from build123d import *

# Parameters (mm, degrees)
F0_R     = 2.5
F1_DEPTH = 5


with BuildPart() as f1:
    # F0 (on Top) → F1 (new body)
    with BuildSketch(Plane.XY):
        with BuildLine():
            ThreePointArc((3.855527, -17.07), (13.669706, -10.926534), (17.5, 0))
            ThreePointArc((17.5, 0), (13.593381, 11.021343), (3.617714, 17.121978))
            ThreePointArc((3.617714, 17.121978), (-0.121713, 17.499577), (-3.855527, 17.07))
            ThreePointArc((-3.855527, 17.07), (-17.499577, -0.121713), (-3.617714, -17.121978))
            ThreePointArc((-3.617714, -17.121978), (0.121713, -17.499577), (3.855527, -17.07))
        make_face()
        Circle(F0_R, mode=Mode.SUBTRACT)
        with BuildLine():
            ThreePointArc((-3.855527, 17.07), (-0.121713, 17.499577), (3.617714, 17.121978))
            Line((3.617714, 17.121978), (3.617714, 19.408765))
            Line((3.617714, 19.408765), (-3.855527, 23.246588))
            Line((-3.855527, 23.246588), (-3.855527, 17.07))
        make_face()
        with BuildLine():
            Line((3.855527, -23.246588), (3.855527, -17.07))
            ThreePointArc((3.855527, -17.07), (0.121713, -17.499577), (-3.617714, -17.121978))
            Line((-3.617714, -17.121978), (-3.617714, -19.408765))
            Line((-3.617714, -19.408765), (3.855527, -23.246588))
        make_face()
    extrude(amount=F1_DEPTH)


solid = f1.part
The listing builds one solid part. Answer for the finished solid, in the listing's coordinates (mm). A direction names the side the tool comes from. Give positions to 0.01 mm unless a question says otherwise; leave off trailing zeros. Loops run counter-clockwise (first coordinate to the right, second up) from the corner with the lowest first, then second, coordinate; pieces in that order, holes last.
Item 1: Determine the mould class of faces 4 (the flat face through (0.067, -21.301, 2.465)), 5 (the flat face through (4, 0, 5)), 6 (the cylindrical face through (-0.54, -2.44, 2.46)) for opening direction X: +X half, -X half, draft (parallel to the pull), parting line (faces both ways), or undercut.
Derived:
face 4: -X half
face 5: draft
face 6: undercut
Item 2: A tool of negligible diameter and unlimited length cuts with its end or side. For faces 1 (the flat face through (3.618, 18, 2)), 2 (the flat face through (-3.618, -18, 2)), 3 (the flat face through (-3.856, 20, 2)), from which of +Z, -Z, +X, -X, +Y, -Y can it reach the whole face along a straight path? Write none if from no direction.
Derived:
face 1: +Z, -Z, +X, +Y
face 2: +Z, -Z, -X, -Y
face 3: +Z, -Z, -X, +Y
Item 3: Find the intervals of material crossed by line 1 along Y through (x, z) = (0, 3); line 2 along X through (y, z) = (19, 3); line 3 along Y through (x, z) = (-12.5, 4), in increasing order.
Derived:
line 1: y = -21.27 to -2.5, 2.5 to 21.27
line 2: x = -3.86 to 3.62
line 3: y = -12.25 to 12.25
Item 4: A cutting plane is placed at B-B (x = 0). Give the vertices of the cut face in (y, z).
Derived:
outline: (-21.27, 0) - (-2.5, 0) - (-2.5, 5) - (-21.27, 5) - close; (2.5, 0) - (21.27, 0) - (21.27, 5) - (2.5, 5) - close
Item 5: Each of these flat-tipped pins is pushed along its axis until it touches: pin 1 Ø1.5 at (y, z) = (-12.5, 4) entering from +X; pin 2 Ø1.5 at (y, z) = (-20.5, 3) entering from +X; pin 3 Ø3 at (y, z) = (-17.5, 4) entering from +X. Where does it stop, or does it pass through?
Derived:
pin 1: stops at x = 12.97
pin 2: stops at x = 3.86
pin 3: stops at x = 7.09
Item 6: A cutting plane is placed at C-C (y = -1.5). Give the vertices of the cut face in (x, z).
Derived:
outline: (-17.44, 0) - (-2, 0) - (-2, 5) - (-17.44, 5) - close; (2, 0) - (17.44, 0) - (17.44, 5) - (2, 5) - close
Item 7: A cutting plane is placed at A-A (z = 1.85). Give the vertices of the cut face in (x, y).
Derived:
outline: (-3.86, 17.07) arc R17.5 ccw to (-3.62, -17.12) - (-3.62, -19.41) - (3.86, -23.25) - (3.86, -17.07) arc R17.5 ccw to (17.5, 0) arc R17.5 ccw to (3.62, 17.12) - (3.62, 19.41) - (-3.86, 23.25) - close; hole circle Ø5 at (0, 0)
Item 8: A cutting plane is placed at D-D (y = 15.5). Give the vertices of the cut face in (x, z).
Derived:
outline: (-8.12, 0) - (8.12, 0) - (8.12, 5) - (-8.12, 5) - close
